The listing builds one solid part. Answer for the finished solid, in the listing's coordinates (mm). A direction names the side the tool comes from. Coordinates: 2 decimals unless noted, no trailing zeros. Loops run counter-clockwise (first coordinate to the right, second up) from the corner with the lowest first, then second, coordinate; pieces in that order, holes last. Notation, with made-up numbers: M -31,50.25 L 7,50.25 A27 ccw 7,82.25 Z; hole C 1.25,-2 d3. An arc over 180 degrees is marked long. Answer in a Markdown table with one row per item. Add a question column.
from build123d import *

# Parameters (mm, degrees)
BOSS_EXTRUDE1_DEPTH             = 179.04999999999998
BOSS_EXTRUDE1_DEPTH_BACK        = 139.19200000000004
BOSS_EXTRUDE2_REACH             = 246.692
BOSS_EXTRUDE2_DIRECTION_2_REACH = 246.692
F_3_8_CLEARANCE_HOLE1_D         = 10.31748
CUT_EXTRUDE1_DEPTH              = 245.69215738419686
CUT_EXTRUDE1_DEPTH_BACK         = 245.69215738419686
FILLET1_R                       = 9.525
CUT_EXTRUDE2_DEPTH              = 101.6
CUT_EXTRUDE2_DEPTH_BACK         = 184.22
FILLET2_START                   = -36
FILLET2_DEPTH                   = 185.025000106
FILLET2_START_2                 = -63.5
FILLET2_2_DEPTH                 = 9.525
FILLET2_START_3                 = 53.975
FILLET2_3_DEPTH                 = 9.525
FILLET2_START_4                 = 149.025000106
FILLET2_4_DEPTH                 = 9.525
FILLET2_5_DEPTH                 = 185.025000106
CUT_EXTRUDE3_DEPTH              = 245.69215738419686
CUT_EXTRUDE3_DEPTH_BACK         = 245.69215738419686
FILLET3_R                       = 9.525
CUT_EXTRUDE4_REACH              = 254.594
CUT_EXTRUDE5_DEPTH              = 245.6921573841969
CUT_EXTRUDE5_DEPTH_BACK         = 25.4
FILLET5_R                       = 9.525
CUT_EXTRUDE6_DEPTH              = 245.6921574759669
CUT_EXTRUDE6_DEPTH_BACK         = 245.6921574759669


with BuildPart() as part:
    # Sketch1 → Boss-Extrude1 (new, two sides: drawn at the far end of the back side and taken through both)
    with BuildSketch(Plane(origin=(0, 0, 0), x_dir=(1, 0, 0), z_dir=(0, 1, 0)).offset(-BOSS_EXTRUDE1_DEPTH_BACK)):
        Polygon((-76.20000000000003, 148.35400023367268), (-76.2000000000001, -12.7), (76.2, -12.7), (76.19999999999997, 148.35400023367268), align=None)
    extrude(amount=BOSS_EXTRUDE1_DEPTH + BOSS_EXTRUDE1_DEPTH_BACK)

    # SurfaceCut1
    split(bisect_by=Plane(origin=(-4.831e-14, -47.89499999999913, 0), x_dir=(1, -6e-17, 0), z_dir=(6e-17, 1, -1.73e-15)), keep=Keep.TOP)

    # Boss-Extrude2: up to this face of the body (flat: up to its plane)
    boss_extrude2_end = Plane(part.part.faces().sort_by_distance((76.2, 65.5775, -67.827000117))[0])
    # Sketch3 → Boss-Extrude2 (add, up to the picked face)
    with BuildSketch(Plane(origin=(0, 0, 0), x_dir=(0, 0, -1), z_dir=(1, 0, 0)), mode=Mode.PRIVATE) as boss_extrude2_sk1:
        Polygon((1.2e-16, -38.36999999999911), (75, -38.36999999999911), (75, -47.89499999999911), (1.29e-15, -47.89499999999911), align=None)
    boss_extrude2_tool1 = split(extrude(boss_extrude2_sk1.sketch, amount=BOSS_EXTRUDE2_REACH, mode=Mode.PRIVATE), bisect_by=boss_extrude2_end, keep=Keep.BOTH, mode=Mode.PRIVATE)
    add(boss_extrude2_tool1.solids().sort_by(Axis((0, -43.1325, -37.5), (1, 0, 0)))[0])

    # Boss-Extrude2 direction 2: up to this face of the body (flat: up to its plane)
    boss_extrude2_direction_2_end = Plane(part.part.faces().sort_by_distance((-76.2, 65.5775, -67.827000117))[0])
    # Sketch3 → Boss-Extrude2 direction 2 (add, up to the picked face)
    with BuildSketch(Plane(origin=(0, 0, 0), x_dir=(0, 0, -1), z_dir=(1, 0, 0)), mode=Mode.PRIVATE) as boss_extrude2_direction_2_sk1:
        Polygon((1.2e-16, -38.36999999999911), (75, -38.36999999999911), (75, -47.89499999999911), (1.29e-15, -47.89499999999911), align=None)
    boss_extrude2_direction_2_tool1 = split(extrude(boss_extrude2_direction_2_sk1.sketch, amount=-BOSS_EXTRUDE2_DIRECTION_2_REACH, mode=Mode.PRIVATE), bisect_by=boss_extrude2_direction_2_end, keep=Keep.BOTH, mode=Mode.PRIVATE)
    add(boss_extrude2_direction_2_tool1.solids().sort_by(Axis((0, -43.1325, -37.5), (-1, 0, 0)))[0])

    # 3/8 Clearance Hole1 (through all)
    with Locations(Plane.XZ.offset(47.89499999999913)):
        with Locations((47.625, -48.895), (-47.625, -48.895), (0, -48.895)):
            Hole(F_3_8_CLEARANCE_HOLE1_D / 2)

    # Sketch8 → Cut-Extrude1 (cut, two sides: drawn at the far end of the back side and taken through both)
    with BuildSketch(Plane(origin=(0, 0, 0), x_dir=(0, 0, -1), z_dir=(1, 0, 0)).offset(-CUT_EXTRUDE1_DEPTH_BACK)):
        Polygon((266.69999999999993, 301.4250001060008), (12.699999999999932, 301.42500010600077), (12.699999999999935, 149.02500010600082), (266.69999999999993, 149.02500010600085), align=None)
    extrude(amount=CUT_EXTRUDE1_DEPTH + CUT_EXTRUDE1_DEPTH_BACK, mode=Mode.SUBTRACT)

    # Fillet1
    fillet1_edges = [part.edges().sort_by_distance(p)[0] for p in [
        (-2.842e-14, 149.02500010600082, -12.699999999999935),
    ]]
    fillet(fillet1_edges, radius=FILLET1_R)

    # Sketch10 → Cut-Extrude2 (cut, two sides: drawn at the far end of the back side and taken through both)
    with BuildSketch(Plane(origin=(0, 149.02500010600082, 1.628e-14), x_dir=(1, 0, 0), z_dir=(0, 1, 1.1e-16)).offset(-CUT_EXTRUDE2_DEPTH_BACK)):
        Polygon((63.500000000000014, 63.49999999999994), (-63.500000000000014, 63.49999999999993), (-63.5, 12.699999999999932), (63.5, 12.699999999999948), align=None)
    extrude(amount=CUT_EXTRUDE2_DEPTH + CUT_EXTRUDE2_DEPTH_BACK, mode=Mode.SUBTRACT)

    # Fillet2: read off the stored shape, not the designer's step
    # Fillet2 outline → Fillet2 (add)
    with BuildSketch(Plane(origin=(0, 0, 0), x_dir=(1, 0, 0), z_dir=(0, 1, 0)).offset(FILLET2_START)):
        with BuildLine():
            Line((-63.5, 12.7), (-53.975, 12.7))
            ThreePointArc((-53.975, 12.7), (-60.710192091, 15.489807909), (-63.5, 22.225))
            Line((-63.5, 22.225), (-63.5, 12.7))
        make_face()
        with BuildLine():
            ThreePointArc((63.5, 22.225), (60.710192091, 15.489807909), (53.975, 12.7))
            Line((53.975, 12.7), (63.5, 12.7))
            Line((63.5, 12.7), (63.5, 22.225))
        make_face()
    extrude(amount=FILLET2_DEPTH)

    # Fillet2 2 outline → Fillet2 2 (add)
    with BuildSketch(Plane.YZ.offset(FILLET2_START_2)):
        with BuildLine():
            Line((149.025000106, -12.7), (149.025000106, -22.225))
            ThreePointArc((149.025000106, -22.225), (151.814808015, -15.489807909), (158.550000106, -12.7))
            Line((158.550000106, -12.7), (149.025000106, -12.7))
        make_face()
    extrude(amount=FILLET2_2_DEPTH)

    # Fillet2 3 outline → Fillet2 3 (add)
    with BuildSketch(Plane.YZ.offset(FILLET2_START_3)):
        with BuildLine():
            Line((149.025000106, -12.7), (149.025000106, -22.225))
            ThreePointArc((149.025000106, -22.225), (151.814808015, -15.489807909), (158.550000106, -12.7))
            Line((158.550000106, -12.7), (149.025000106, -12.7))
        make_face()
    extrude(amount=FILLET2_3_DEPTH)

    # Fillet2 4 outline → Fillet2 4 (cut)
    with BuildSketch(Plane(origin=(0, 0, 0), x_dir=(1, 0, 0), z_dir=(0, 1, 0)).offset(FILLET2_START_4)):
        with BuildLine():
            Line((-53.975, 22.225), (-63.5, 22.225))
            ThreePointArc((-63.5, 22.225), (-60.710192091, 15.489807909), (-53.975, 12.7))
            Line((-53.975, 12.7), (-53.975, 22.225))
        make_face()
        with BuildLine():
            ThreePointArc((53.975, 12.7), (60.710192091, 15.489807909), (63.5, 22.225))
            Line((63.5, 22.225), (53.975, 22.225))
            Line((53.975, 22.225), (53.975, 12.7))
        make_face()
    extrude(amount=FILLET2_4_DEPTH, mode=Mode.SUBTRACT)

    # Fillet2 5 outline → Fillet2 5 (add)
    with BuildSketch(Plane(origin=(0, 0, 0), x_dir=(1, 0, 0), z_dir=(0, 1, 0)).offset(FILLET2_START)):
        with BuildLine():
            ThreePointArc((53.975, 63.5), (60.710192091, 60.710192091), (63.5, 53.975))
            Line((63.5, 53.975), (63.5, 22.225))
            Line((63.5, 22.225), (76.2, 22.225))
            Line((76.2, 22.225), (76.2, 148.354000234))
            Line((76.2, 148.354000234), (-76.2, 148.354000234))
            Line((-76.2, 148.354000234), (-76.2, 22.225))
            Line((-76.2, 22.225), (-63.5, 22.225))
            Line((-63.5, 22.225), (-63.5, 53.975))
            ThreePointArc((-63.5, 53.975), (-60.710192091, 60.710192091), (-53.975, 63.5))
            Line((-53.975, 63.5), (53.975, 63.5))
        make_face()
    extrude(amount=FILLET2_5_DEPTH)

    # Sketch11 → Cut-Extrude3 (cut, two sides: drawn at the far end of the back side and taken through both)
    with BuildSketch(Plane(origin=(0, 0, 0), x_dir=(0, 0, -1), z_dir=(1, 0, 0)).offset(-CUT_EXTRUDE3_DEPTH_BACK)):
        Polygon((279.3999999999999, 413.26880624754574), (76.19999999999999, -22.494999999999397), (76.19999999999999, -78.83303235544759), (279.3999999999999, -78.83303235544756), align=None)
    extrude(amount=CUT_EXTRUDE3_DEPTH + CUT_EXTRUDE3_DEPTH_BACK, mode=Mode.SUBTRACT)

    # Fillet3
    fillet3_edges = [part.edges().sort_by_distance(p)[0] for p in [
        (-5.684e-14, -22.494999999999397, -76.19999999999999),
    ]]
    fillet(fillet3_edges, radius=FILLET3_R)

    # Cut-Extrude4: up to this face of the body (flat: up to its plane)
    cut_extrude4_end = Plane(part.part.faces().sort_by_distance((0, 75.599563928, -12.7))[0])
    # Sketch14 → Cut-Extrude4 (cut, up to the picked face)
    with BuildSketch(Plane(origin=(0, 0, -148.35400023367268), x_dir=(-1, 0, 0), z_dir=(0, 0, -1)), mode=Mode.PRIVATE) as cut_extrude4_sk1:
        Polygon((-63.5, 136.32500010600086), (63.5, 136.32500010600089), (63.50000000000004, -35.19499999999937), (-63.499999999999986, -35.19499999999938), align=None)
    cut_extrude4_tool1 = split(extrude(cut_extrude4_sk1.sketch, amount=-CUT_EXTRUDE4_REACH, mode=Mode.PRIVATE), bisect_by=cut_extrude4_end, keep=Keep.BOTH, mode=Mode.PRIVATE)
    add(cut_extrude4_tool1.solids().sort_by(Axis((0, 50.565, -148.354), (0, 0, 1)))[0], mode=Mode.SUBTRACT)

    # Sketch15 → Cut-Extrude5 (cut, two sides: drawn at the far end of the back side and taken through both)
    with BuildSketch(Plane.XY.offset(-CUT_EXTRUDE5_DEPTH_BACK)):
        Polygon((63.5, 159.99999999999997), (-63.5, 159.99999999999994), (-63.500000000000014, -35.194999999999425), (63.50000000000007, -35.19499999999941), align=None)
    extrude(amount=CUT_EXTRUDE5_DEPTH + CUT_EXTRUDE5_DEPTH_BACK, mode=Mode.SUBTRACT)

    # Fillet5
    fillet5_edges = [part.edges().sort_by_distance(p)[0] for p in [
        (63.5, 159.99999999999997, 2.842e-14),
        (-63.5, 159.99999999999994, 2.842e-14),
        (-63.5, 136.32500010600089, -101.16450011683634),
        (63.5, 136.32500010600086, -101.16450011683634),
        (63.5, -35.19499989399918, -38.1),
        (-63.5, -35.19499989399918, -38.1),
    ]]
    fillet(fillet5_edges, radius=FILLET5_R)

    # Sketch16 → Cut-Extrude6 (cut, two sides: drawn at the far end of the back side and taken through both)
    with BuildSketch(Plane(origin=(0, 0, 0), x_dir=(0, 0, -1), z_dir=(1, 0, 0)).offset(-CUT_EXTRUDE6_DEPTH_BACK)):
        with BuildLine():
            Line((22.225, -20.152543088136632), (43.61046140315716, -20.152543088136635))
            ThreePointArc((43.61046140315716, -20.152543088136635), (48.871667611787636, -18.266432044059904), (52.27951237608929, -13.836499798218902))
            Line((52.27951237608929, -13.836499798218902), (110.28947349119366, 110.6974636611936))
            ThreePointArc((110.28947349119366, 110.6974636611936), (109.2394256542931, 119.49983646292918), (101.39293648279772, 123.62500010600078))
            Line((101.39293648279772, 123.62500010600078), (22.225000000000072, 123.6250001060008))
            ThreePointArc((22.225000000000072, 123.6250001060008), (15.489807909198145, 120.83519219680267), (12.700000000000001, 114.10000010600075))
            Line((12.700000000000001, 114.10000010600075), (12.7, -10.627543088136633))
            ThreePointArc((12.7, -10.627543088136633), (15.489807909198138, -17.362735178938497), (22.225, -20.152543088136632))
        make_face()
    extrude(amount=CUT_EXTRUDE6_DEPTH + CUT_EXTRUDE6_DEPTH_BACK, mode=Mode.SUBTRACT)


solid = part.part
(1) For faces 1 (the face through (-1, 149.025, -98)), 2 (the face through (-60.784, -32.331, -32.372)), 3 (the face through (-69.939, 119.393, -109.312)), 4 (the face through (1, 143, -63.5)), determine the directions among +Z, -Z, +X, -X, +Y, -Y from which every point of the face is accessible in a straight line to the end or side of a thin tool.
(2) Each of these flat-tipped pins is pushed along its axis until it touches: pin 1 (16.5 mm diameter, centred on x = 47.625, z = -48.895, fed in from +Y); pin 2 (14 mm diameter, centred on x = -67, z = -29.5, fed in from +Y) (3 decimals); pin 3 (6 mm diameter, centred on x = -10, y = 165.5, fed in from -Z); pin 4 (9.5 mm diameter, centred on x = 0, z = -48.895, fed in from +Y). Where does it stop, or does it pass through?
(3) A cutting plane is placed at A-A (x = -28.5). Give the vertices of the cut face in (y, z) (3 decimals), plus the area to 3 significant figures.
(4) The mould has two halves that part along X. Classify faces 5 (the face through (69.761, 119.393, -109.312)), 6 (the face through (61.72, 140.23, -59.52)): released by +X, released by -X, zero draft, split by the parting line, or undercut.
(5) A cutting plane is placed at D-D (y = -3). Give the vertices of the cut face in (x, z).
(6) Straight lines are drawn through the part: line 1 (Y direction, x = -48.5, z = -5) (3 decimals); line 2 (Z direction, x = 0, y = -45); line 3 (Y direction, x = 52.5, z = -70) (3 decimals). For each, find the intervals that lie inside material, in ascending order.
(7) A cutting plane is placed at B-B (z = -8). Give the vertices of the cut face in (x, y) (3 decimals), plus the area to 3 significant figures.
(8) A cutting plane is placed at C-C (x = 0). Give the vertices of the cut face in (y, z) (3 decimals).
Solved:
| question | item | result |
|---|---|---|
| 1 | face 1 | -Z, +X, -X, +Y |
| 1 | face 2 | +Z, -Z |
| 1 | face 3 | +X, -X |
| 1 | face 4 | +Z, +Y |
| 2 | pin 1 | stops at y = -35 |
| 2 | pin 2 | stops at y = 149.025 |
| 2 | pin 3 | stops at z = -12.7 |
| 2 | pin 4 | passes through |
| 3 | outline | M -47.895,-76.2 L -35.195,-76.2 L -35.195,12.7 L -47.895,12.7 Z; M 136.325,-148.354 L 149.025,-148.354 L 149.025,-63.5 L 136.325,-63.5 Z; M 160,-12.7 L 179.05,-12.7 L 179.05,12.7 L 160,12.7 Z |
| 3 | area | 2,690 mm² |
| 4 | face 5 | zero draft |
| 4 | face 6 | undercut |
| 5 | outline | M -76.2,-85.29 L -63.5,-85.29 L -63.5,-57.33 L -76.2,-57.33 Z; M -76.2,-12.7 L -63.5,-12.7 L -63.5,12.7 L -76.2,12.7 Z; M 63.5,-85.29 L 76.2,-85.29 L 76.2,-57.33 L 63.5,-57.33 Z; M 63.5,-12.7 L 76.2,-12.7 L 76.2,12.7 L 63.5,12.7 Z |
| 6 | line 1 | y = -47.895 to -35.195, 160 to 179.05 |
| 6 | line 2 | z = -76.2 to -54.05, -43.74 to 12.7 |
| 6 | line 3 | y = -47.895 to -35.195, 136.325 to 149.025 |
| 7 | outline | M -76.2,-47.895 L 76.2,-47.895 L 76.2,179.05 L -76.2,179.05 Z; hole M -63.5,-25.67 A9.525 ccw -53.975,-35.195 L 53.975,-35.195 A9.525 ccw 63.5,-25.67 L 63.5,150.475 A9.525 ccw 53.975,160 L -53.975,160 A9.525 ccw -63.5,150.475 Z |
| 7 | area | 9,870 mm² |
| 8 | outline | M -47.895,-76.2 L -35.195,-76.2 L -35.195,-54.054 L -47.895,-54.054 Z; M -47.895,-43.736 L -35.195,-43.736 L -35.195,12.7 L -47.895,12.7 Z; M 136.325,-148.354 L 149.025,-148.354 L 149.025,-63.5 L 136.325,-63.5 Z; M 160,-12.7 L 179.05,-12.7 L 179.05,12.7 L 160,12.7 Z |
